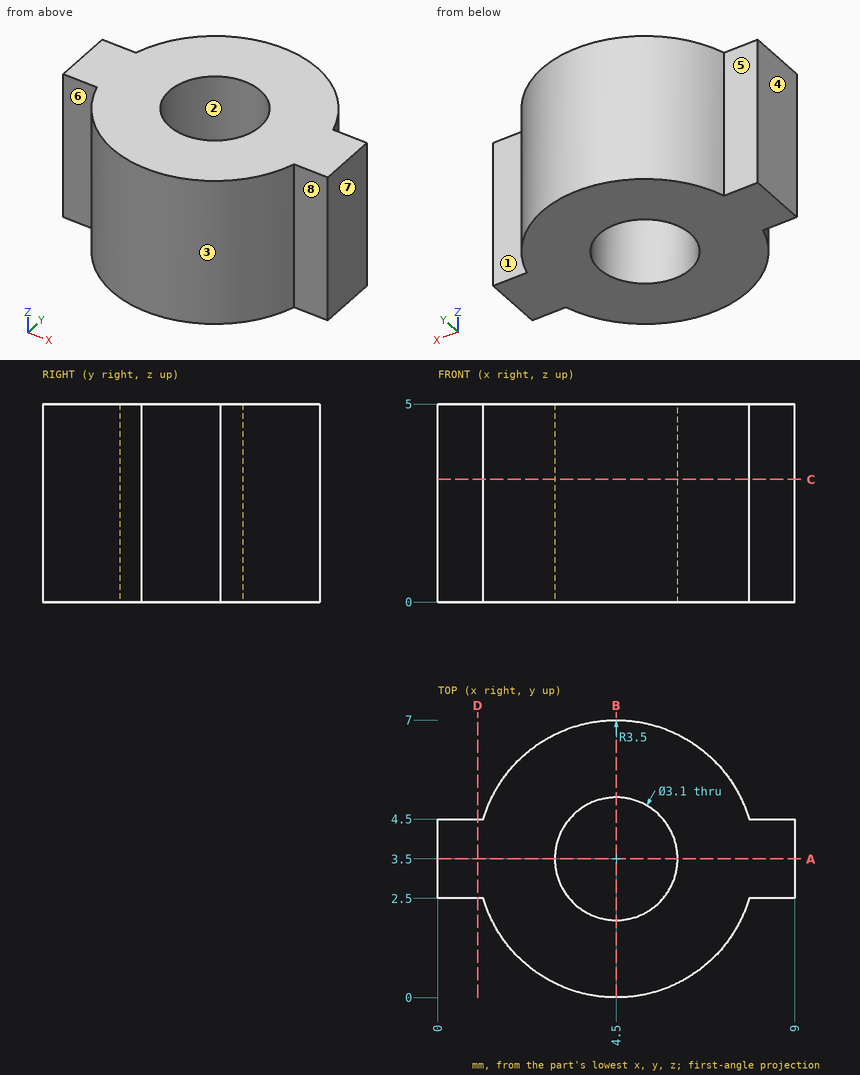
Geometry check sheet. Reference: drawing and pictorial views, mm from the part's lowest x, y, z. A direction names the side the tool comes from. Round coordinates to 2 decimals unless told otherwise and drop trailing zeros. Order: outer loops, then holes, each group sorted by start corner. A loop starts at its lowest first (then second) coordinate and runs counter-clockwise, first axis right, second up. Notation, with made-up numbers: M 59,39 L 110,39 A23 ccw 110,53 Z; hole C 3,15.5 d4. An arc over 180 degrees is marked long. One line per item, written item: value. Start each with the question number.
1. Release check for a two-part mould opening along Y. For the marked faces 1, 2, 3 and 4 record: released by +Y, released by -Y, zero draft, split by the parting line, or undercut.
2. Section check B-B on x = 4.5. Enter the section's corners in (y, z).
3. Section check A-A on y = 3.5. Enter the section's corners in (x, z).
4. Access from +Z, -Z, +X, -X, +Y, -Y to the whole of each face (thin tool, end or side, straight path). Record for the marked faces 5, 6, 7 and 8.
5. Scan lines: line 1 along Y through (x, z) = (4.5, 3.25); line 2 along X through (y, z) = (2.25, 1.35); line 3 along X through (y, z) = (1.25, 4.2). Record each from-to range of solid material in increasing order.
6. Gauge pin test, flat ends, axial feed: P1, Ø3, axis at y = 5.5, z = 1, coming from the -X side; P2, Ø0.6, axis at x = 0.5, z = 2, coming from the +Y side; P3, Ø0.6, axis at x = 8.5, z = 1.5, coming from the -Y side. Record the tip position at first contact, or that the pin passes through.
7. Section check C-C on z = 3.1. Enter the section's corners in (x, y), and give its area (3 significant figures).
8. Section check D-D on x = 1. Enter the section's corners in (y, z).
Results found:
1. face 1: released by +Y
1. face 2: undercut
1. face 3: released by -Y
1. face 4: zero draft
2. outline: M 0,0 L 1.95,0 L 1.95,5 L 0,5 Z; M 5.05,0 L 7,0 L 7,5 L 5.05,5 Z
3. outline: M 0,0 L 2.95,0 L 2.95,5 L 0,5 Z; M 6.05,0 L 9,0 L 9,5 L 6.05,5 Z
4. face 5: +Z, -Z, -X, +Y
4. face 6: +Z, -Z, -X, -Y
4. face 7: +Z, -Z, +X, +Y, -Y
4. face 8: +Z, -Z, +X, -Y
5. line 1: 0 to 1.95, 5.05 to 7
5. line 2: 1.23 to 3.58, 5.42 to 7.77
5. line 3: 1.82 to 7.18
6. P1: x = 0
6. P2: y = 4.5
6. P3: y = 2.5
7. outline: M 0,2.5 L 1.15,2.5 A3.5 ccw 7.85,2.5 L 9,2.5 L 9,4.5 L 7.85,4.5 A3.5 ccw 1.15,4.5 L 0,4.5 Z; hole C 4.5,3.5 d3.1
7. area: 35.1 mm^2
8. outline: M 2.5,0 L 4.5,0 L 4.5,5 L 2.5,5 Z
